For this review, use the dimensioned drawing (mm, ordinates from the lowest corner) and the shaded views. A direction names the side the tool comes from. Coordinates: 2 decimals unless noted, no trailing zeros. Write each loop counter-clockwise with the first axis right and the second up, starting at its lowest first coordinate (ties: lowest second). Pieces come first, ordered by that corner, then holes. Notation, with made-up numbers: M 43.5,13 L 74.5,13 A28 ccw 74.5,44 Z; hole C 84,34.25 d9. An arc over 180 degrees is marked long. Return JSON: item names as keys, results as strings. Group by question number.
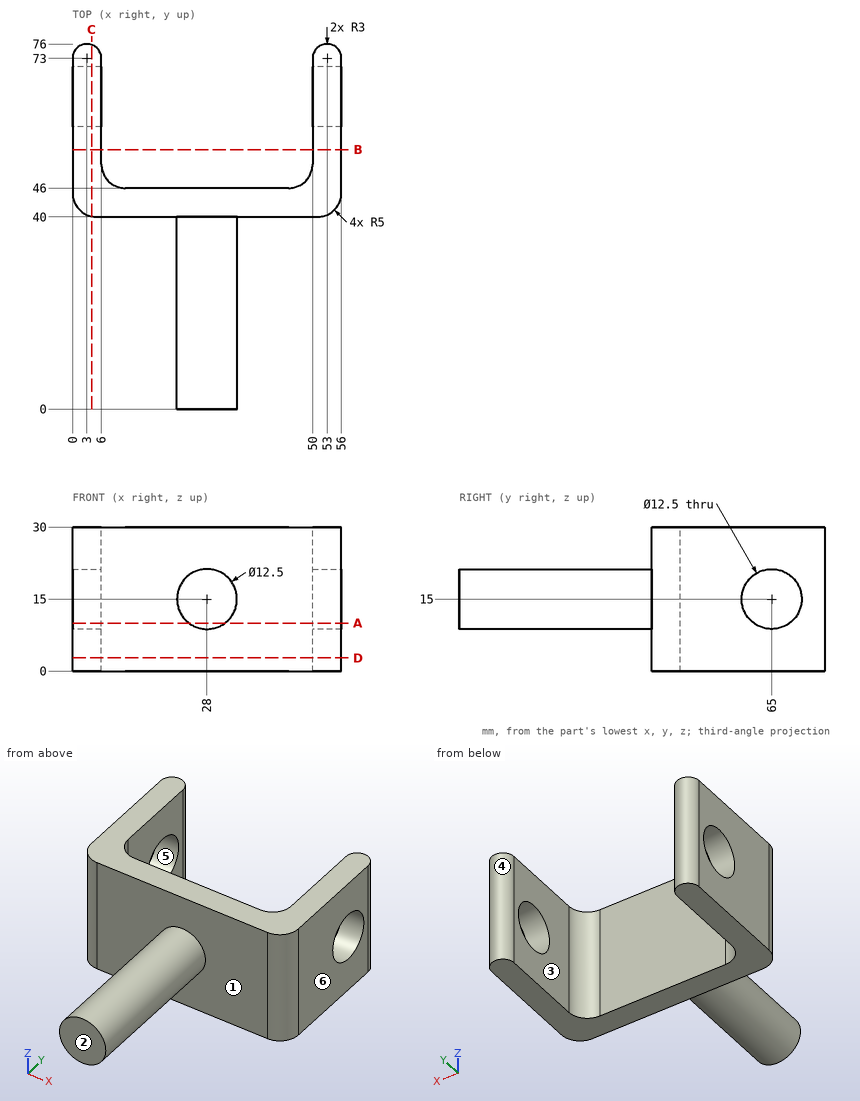
Item 1: For line 1 (X direction, y = 62.5, z = 3); line 2 (Y direction, x = 11.5, z = 5); line 3 (Y direction, x = 26.5, z = 9), list the stretches that pass through material, from the lowest coordinate up.
Item 2: Machinability: for the marked faces 1, 2 and 3, which of the approach directions +Z, -Z, +X, -X, +Y, -Y give a long, thin tool a straight path to every point of the face, cutting with its end or side? Answer none if there is none.
Item 3: Add section C-C (x = 4). Write out the cut boundary in (y, z), plus the area to 3 significant figures.
Item 4: For pin 1 (2 mm diameter, centred on y = 15.5, z = 7.5, fed in from -X); pin 2 (5 mm diameter, centred on x = 35.5, z = 10, fed in from +Y); pin 3 (1.5 mm diameter, centred on y = 41, z = 10.5, fed in from +X); pin 4 (3 mm diameter, centred on x = 8, z = 24.5, fed in from +Y), all flat-tipped, find the tip position at first contact; note any pin that passes through.
Item 5: Add section B-B (y = 54). Write out the cut boundary in (x, z), plus the area to 3 significant figures.
Item 6: Add section D-D (z = 2.75). Write out the cut boundary in (x, y).
Item 7: Add section A-A (z = 10). Write out the cut boundary in (x, y).
Item 8: The part is to be moulded in two halves that separate along Y. For the marked faces 4, 5 and 6, say which applies: pulls with the +Y half, pulls with the -Y half, needs draft (parallel to the pull), parting line crosses it, or undercut.
Geometry check:
{
 "1": {"line 1": "0 to 6, 50 to 56", "line 2": "40 to 46", "line 3": "0 to 46"},
 "2": {"face 1": "-Y", "face 2": "+Z, -Z, +X, -X, -Y", "face 3": "+Z, -Z, +Y"},
 "3": {"outline": "M 40.1,0 L 75.83,0 L 75.83,30 L 40.1,30 Z; hole C 65,15 d12.5", "area": "949 mm^2"},
 "4": {"pin 1": "through", "pin 2": "y = 46", "pin 3": "x = 54.8", "pin 4": "y = 48.82"},
 "5": {"outline": "M 0,0 L 6,0 L 6,30 L 0,30 Z; M 50,0 L 56,0 L 56,30 L 50,30 Z", "area": "360 mm^2"},
 "6": {"outline": "M 0,45 A5 ccw 5,40 L 51,40 A5 ccw 56,45 L 56,73 A3 ccw 50,73 L 50,51 A5 cw 45,46 L 11,46 A5 cw 6,51 L 6,73 A3 ccw 0,73 Z"},
 "7": {"outline": "M 0,45 A5 ccw 5,40 L 24.25,40 L 24.25,0 L 31.75,0 L 31.75,40 L 51,40 A5 ccw 56,45 L 56,61.25 L 50,61.25 L 50,51 A5 cw 45,46 L 11,46 A5 cw 6,51 L 6,61.25 L 0,61.25 Z; M 0,68.75 L 6,68.75 L 6,73 A3 ccw 0,73 Z; M 50,68.75 L 56,68.75 L 56,73 A3 ccw 50,73 Z"},
 "8": {"face 4": "pulls with the +Y half", "face 5": "undercut", "face 6": "needs draft"}
}
